Here's how the part is built. I have some questions about the finished solid (model axes, mm). Round coordinates to 2 decimals unless told otherwise and drop trailing zeros. Write each loop counter-clockwise with the first axis right and the second up, starting at its lowest first coordinate (ties: lowest second). Pieces come first, ordered by that corner, then holes. Notation, with made-up numbers: (37.5, 59.5) -> (56.5, 59.5) arc R6 cw to (56.5, 64.5) -> close; hole circle Ø7 at (78, 14). An arc over 180 degrees is marked (long way). Answer in a Markdown table with one row per item. Add a question column.
from build123d import *

# Parameters (mm, degrees)
F0_W     = 200
F0_H     = 100
F1_DEPTH = 30
F2_SIZE2 = 10
F2_SIZE  = 10


with BuildPart() as f1:
    # F0 (on Front) → F1 (new body)
    with BuildSketch(Plane.XZ):
        Rectangle(F0_W, F0_H)
    extrude(amount=F1_DEPTH)

    # F2
    f2_edges = [f1.edges().sort_by_distance(p)[0] for p in [
        (0, -30, 50),
        (0, -30, -50),
        (100, -30, 0),
        (-100, -30, 0),
        (-100, 0, 0),
        (0, 0, 50),
        (0, 0, -50),
        (100, 0, 0),
    ]]
    chamfer(f2_edges, length=F2_SIZE, length2=F2_SIZE2)


solid = f1.part
Item 1: If we section it at B-B on z = 2: Please give me the cut outline in (x, y).
Item 2: For P1, Ø3, axis at y = -9, z = 31, coming from the +X side; P2, Ø5, axis at x = 59.5, y = -5, coming from the -Z side; P3, Ø3, axis at y = -6, z = 14.5, coming from the -X side, each with a flat end and sliding along its axis, tell me the tip position at first contact or that it passes through.
Item 3: If we section it at C-C on y = -3: Please give me the cut outline in (x, z), then the cut area to 3 significant figures.
Item 4: I need wall thicknesses on line 1 along X through (y, z) = (-7.5, -15.5); line 2 along Z through (x, y) = (53.5, -8); line 3 along Z through (x, y) = (-54, -24). Which ranges of each line are inside material? Lowest first, please. Write a range as from..to.
Item 5: If we section it at A-A on x = 15: Please give me the cut outline in (y, z), then the cut area to 3 significant figures.
Item 6: If we section it at D-D on y = -28: Please give me the cut outline in (x, z).
Results list:
| question | item | result |
|---|---|---|
| 1 | outline | (-100, -20) -> (-90, -30) -> (90, -30) -> (100, -20) -> (100, -10) -> (90, 0) -> (-90, 0) -> (-100, -10) -> close |
| 2 | P1 | x = 100 |
| 2 | P2 | z = -47.5 |
| 2 | P3 | x = -97.5 |
| 3 | outline | (-93, -43) -> (93, -43) -> (93, 43) -> (-93, 43) -> close |
| 3 | area | 16,000 mm² |
| 4 | line 1 | -97.5..97.5 |
| 4 | line 2 | -48..48 |
| 4 | line 3 | -46..46 |
| 5 | outline | (-30, -40) -> (-20, -50) -> (-10, -50) -> (0, -40) -> (0, 40) -> (-10, 50) -> (-20, 50) -> (-30, 40) -> close |
| 5 | area | 2,800 mm² |
| 6 | outline | (-92, -42) -> (92, -42) -> (92, 42) -> (-92, 42) -> close |
